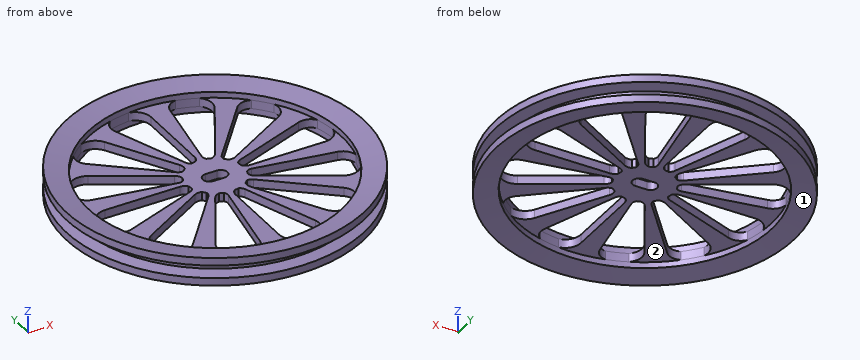
from build123d import *

# Parameters (mm, degrees)
CUT_EXTRUDE3_START = -2.387057914
CUT_EXTRUDE3_DEPTH = 2.387057914
CIRPATTERN2_COUNT  = 12
CUT_EXTRUDE4_DEPTH = 59.793512223


# Read off the part's stored shape, not the designer's step: Cut-Extrude3
with BuildPart() as part:
    # Sketch1 → Revolve1 (revolve)
    with BuildSketch(Plane(origin=(0, 0, 0), x_dir=(0, 0, -1), z_dir=(1, 0, 0)), mode=Mode.PRIVATE) as revolve1_sk:
        Polygon((-1.193528957, 0), (-1.193528957, 35.218988836), (-2.844528957, 35.218988836), (-3.937, 41.4147), (-1.778, 41.4147), (-1.193528957, 38.1), (1.193528957, 38.1), (1.778, 41.4147), (3.937, 41.4147), (2.844528957, 35.218988836), (1.193528957, 35.218988836), (1.193528957, 0), align=None)
    revolve(revolve1_sk.sketch.rotate(Axis((0, 0, 1.193528957), (0, 0, -1)), 180), axis=Axis((0, 0, 1.193528957), (0, 0, -1)))

    # Cut-Extrude3 outline → Cut-Extrude3 (cut)
    with BuildSketch(Plane(origin=(0, 0, -1.193528957), x_dir=(-1, 0, 0), z_dir=(0, 0, -1)).offset(CUT_EXTRUDE3_START)):
        with BuildLine():
            ThreePointArc((2.066345579, 7.663819035), (2.76104062, 8.106910335), (3.203637142, 8.801920708))
            Line((3.203637142, 8.801920708), (10.751653826, 29.539926109))
            ThreePointArc((10.751653826, 29.539926109), (10.809621103, 31.974229594), (9.381543944, 33.946484469))
            ThreePointArc((9.381543944, 33.946484469), (6.561048987, 34.602453827), (3.696198494, 35.02449559))
            ThreePointArc((3.696198494, 35.02449559), (1.047467977, 33.509168244), (0, 30.643020803))
            Line((0, 30.643020803), (0, 9.811006208))
            ThreePointArc((0, 9.811006208), (0.230432564, 8.753888306), (0.879919889, 7.88857701))
            ThreePointArc((0.879919889, 7.88857701), (1.477412972, 7.798792032), (2.066345579, 7.663819035))
        make_face()
    cut_extrude3 = extrude(amount=CUT_EXTRUDE3_DEPTH, mode=Mode.SUBTRACT)

    # CirPattern2: Cut-Extrude3 ×12 about axis
    cirpattern2_axis = Axis((0, 0, 0), (0, 0, 1))
    for i in range(1, CIRPATTERN2_COUNT):
        add(cut_extrude3.rotate(cirpattern2_axis, i * 360 / CIRPATTERN2_COUNT), mode=Mode.SUBTRACT)

    # Sketch2 → Cut-Extrude4 (cut, through all)
    with BuildSketch(Plane(origin=(0, 0, -1.193528957), x_dir=(-1, 0, 0), z_dir=(0, 0, -1))):
        with BuildLine():
            Line((-1.5875, 1.8415), (1.5875, 1.8415))
            ThreePointArc((1.5875, 1.8415), (3.429, 0), (1.5875, -1.8415))
            Line((1.5875, -1.8415), (-1.5875, -1.8415))
            ThreePointArc((-1.5875, -1.8415), (-3.429, 0), (-1.5875, 1.8415))
        make_face()
    extrude(amount=-CUT_EXTRUDE4_DEPTH, mode=Mode.SUBTRACT)


solid = part.part
Work out the finished part from the listing and answer in its coordinate system (mm). Face numbers are marked on the shaded views. Coordinates: 2 decimals unless noted, no trailing zeros. Put each result on its own line as item: value. Start each with the question number.
1) For a pull along Y with two mould halves and no side action, classify the marked faces 1 and 2 as released by +Y, released by -Y, zero draft, split by the parting line, or undercut.
2) Find the intervals of material crossed by line 1 (X direction, y = 0, z = 2.5); line 2 (X direction, y = 24, z = -0.5); line 3 (Y direction, x = -13.5, z = 1), in increasing order. Write a range as from..to.
3) Flat-ended cylindrical pins translate along their axes: pin 1 (6 mm diameter, centred on x = 10.5, y = -30, fed in from +Z); pin 2 (1 mm diameter, centred on x = -19.5, y = -31, fed in from +Z); pin 3 (1.5 mm diameter, centred on x = -2, z = -2, fed in from -Y). Find the tip coordinate at first contact, or state that the pin passes through.
Results list:
1. face 1: undercut
1. face 2: undercut
2. line 1: x = -41.41..-35.22, 35.22..41.41
2. line 2: x = -29.59..-25.34, -13.86..-8.74, 0..4.23, 13.86..20.14, 25.78..29.59
2. line 3: y = -35.63..-32.53, -23.38..-16.09, -7.79..-4.91, 0..2.38, 7.79..11.33, 23.38..35.63
3. pin 1: stops at z = 1.19
3. pin 2: stops at z = 3.18
3. pin 3: stops at y = -41.4
